```python
from build123d import *

# Parameters (mm, degrees)
F3_ANGLE = 167
F4_SIZE  = 1


# Not quite as in the source:
# - a feature names something its author has since deleted; it is built from what else it names


with BuildPart() as f3:
    # F2 (on Front) → F3 (revolve)
    with BuildSketch(Plane.XZ):
        Polygon((-753.25, 20), (-756.75, 20), (-756.75, 0), (-735.25, 0), (-735.25, 3.5), (-753.25, 3.5), align=None)
    revolve(axis=Axis((0, 0, 7.6849460602), (0, 0, -1)), revolution_arc=F3_ANGLE)

    # F4
    f4_edges = [f3.edges().sort_by_distance(p)[0] for p in [
        (-85.666532, 751.885502, 20),
        (-85.270321, 748.408, 20),
    ]]
    chamfer(f4_edges, length=F4_SIZE)


solid = f3.part
```
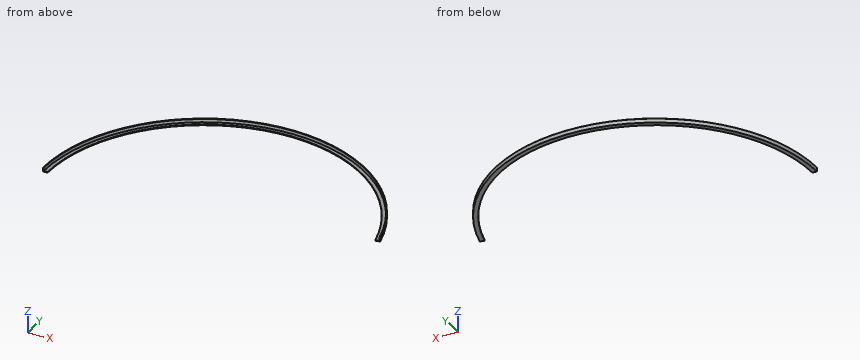
Here's how the part is built. I have some questions about the finished solid (model axes, mm). Coordinates: 2 decimals unless noted, no trailing zeros. Order: outer loops, then holes, each group sorted by start corner. A loop starts at its lowest first (then second) coordinate and runs counter-clockwise, first axis right, second up.
1) Will these pins go through, and if not, where does the flat tip stop? pin 1 (10 mm diameter, centred on y = 396.5, z = 7, fed in from +X); pin 2 (6 mm diameter, centred on x = 407, z = 3, fed in from -Y); pin 3 (5 mm diameter, centred on x = 93, z = 9.5, fed in from +Y).
2) Imagine slicing it at A-A on z = 8. List the corners of the cut face in (x, y) for me, and give its area (3 significant figures).
3) I need wall thicknesses on line 1 (X direction, y = 664, z = 2); line 2 (X direction, y = 538, z = 3.75); line 3 (X direction, y = 64, z = 2.75). Which ranges of each line are inside material? Lowest first, please.
Response values:
1. pin 1: stops at x = 647.61
1. pin 2: stops at y = 610.32
1. pin 3: stops at y = 751.32
2. outline: (-756.75, 0) - (-753.25, 0) arc R753.25 cw to (733.94, 169.44) - (737.35, 170.23) arc R756.75 ccw to start
2. area: 7,700 mm2
3. line 1: x = -363.01 to -315.75, 315.75 to 363.01
3. line 2: x = -532.19 to -527.2, 527.2 to 532.19
3. line 3: x = -754.04 to -732.46
